Study the drawing (mm; zero at the part's minimum x, y, z) and answer. Round coordinates to 2 decimals unless told otherwise and drop trailing zeros. Write each loop counter-clockwise with the first axis right and the second up, starting at its lowest first coordinate (ties: lowest second). Pieces come first, ordered by that corner, then holes.
(1) Each of these flat-tipped pins is pushed along its axis until it touches: pin 1 Ø7 at (x, z) = (19, 63) entering from -Y; pin 2 Ø2 at (x, z) = (8, 30.5) entering from -Y (3 decimals); pin 3 Ø12 at (x, z) = (10, 82.5) entering from -Y. Where does it stop, or does it pass through?
(2) A cutting plane is placed at C-C, the plane x = 21.5. Give the vertices of the cut face in (y, z) (1 decimal), and give its area (3 significant figures).
(3) A cutting plane is placed at B-B, the plane y = 7. Give the vertices of the cut face in (x, z), and give its area (3 significant figures).
(4) Find the intervals of material crossed by probe 1 along Z at (x, y) = (18, 9.5); probe 2 along Y at (x, z) = (4.5, 34.5) (1 decimal); probe 3 along Z at (x, y) = (16.51, 23.5) (3 decimals), in increasing order.
(5) The mould has two halves that part along Y. Classify the marked faces 1, 2 and 3: +Y half, -Y half, draft (parallel to the pull), parting line (faces both ways), or undercut.
(6) A cutting plane is placed at D-D, the plane z = 48. Give the vertices of the cut face in (x, y) (1 decimal).
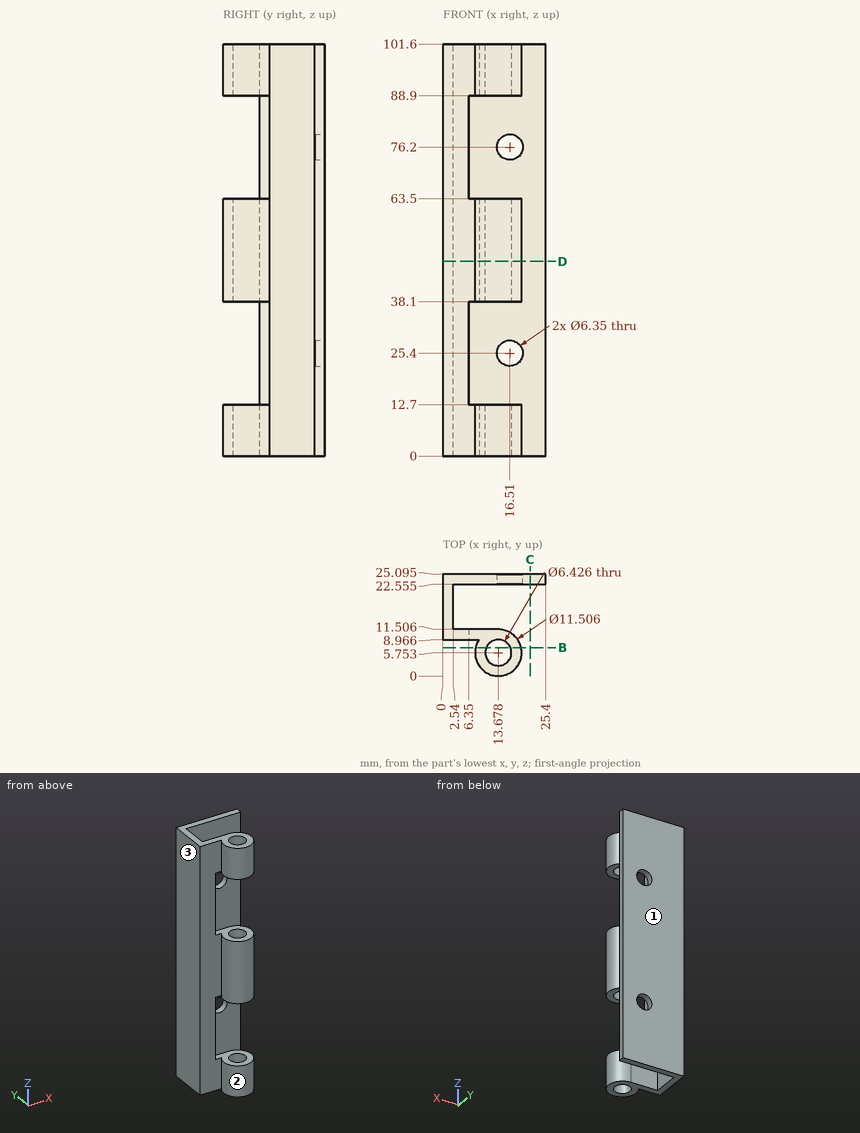
Solutions:
1. pin 1: stops at y = 0.3
1. pin 2: stops at y = 22.555
1. pin 3: stops at y = 8.97
2. outline: (22.6, 0) - (25.1, 0) - (25.1, 101.6) - (22.6, 101.6) - close
2. area: 258 mm2
3. outline: (8.06, 0) - (10.72, 0) - (10.72, 12.7) - (8.06, 12.7) - close; (8.06, 38.1) - (10.72, 38.1) - (10.72, 63.5) - (8.06, 63.5) - close; (8.06, 88.9) - (10.72, 88.9) - (10.72, 101.6) - (8.06, 101.6) - close; (16.64, 0) - (19.29, 0) - (19.29, 12.7) - (16.64, 12.7) - close; (16.64, 38.1) - (19.29, 38.1) - (19.29, 63.5) - (16.64, 63.5) - close; (16.64, 88.9) - (19.29, 88.9) - (19.29, 101.6) - (16.64, 101.6) - close
3. area: 270 mm2
4. probe 1: z = 0 to 12.7, 38.1 to 63.5, 88.9 to 101.6
4. probe 2: y = 9 to 11.5, 22.6 to 25.1
4. probe 3: z = 0 to 22.225, 28.575 to 73.025, 79.375 to 101.6
5. face 1: +Y half
5. face 2: undercut
5. face 3: draft
6. outline: (0, 9) - (8.9, 9) arc R5.8 ccw (long way) to (13.7, 11.5) - (2.5, 11.5) - (2.5, 22.6) - (25.4, 22.6) - (25.4, 25.1) - (0, 25.1) - close; hole circle Ø6.4 at (13.7, 5.8)
